Input: dimensioned drawing with shaded views. Units: mm. Origin: part minimum x, y, z. Coordinates: 2 decimals unless noted, no trailing zeros. Order: outer loops, then holes, each group sorted by start corner. A loop starts at its lowest first (then second) coordinate and runs counter-clockwise, first axis right, second up. Notation, with made-up numbers: (34.25, -3) -> (44.25, -3) arc R21 cw to (44.25, 16) -> close; hole circle Ø1 at (-1, 64.5). An arc over 180 degrees is marked (long way). Put each result on its own line as item: value.
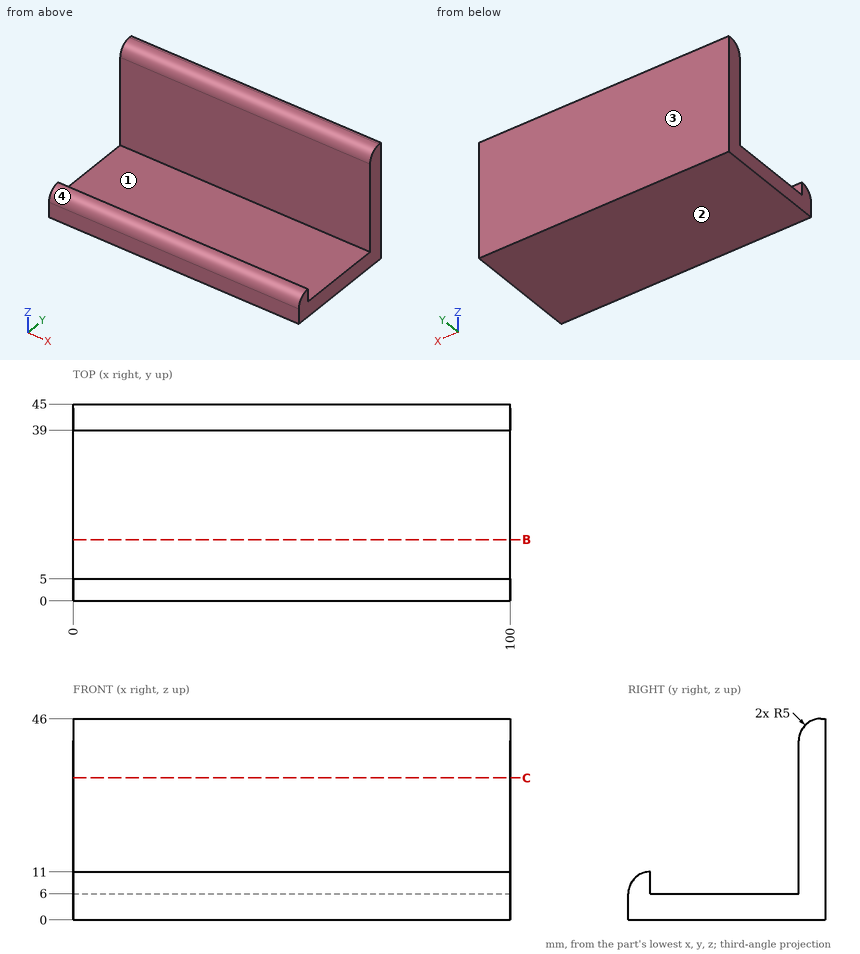
1. Cut plane C-C on z = 32.5. Output: boundary loops of the cut face in (x, y).
Numbers:
outline: (0, 39) -> (100, 39) -> (100, 45) -> (0, 45) -> close
2. Cut plane B-B on y = 14. Output: boundary loops of the cut face in (x, z).
Numbers:
outline: (0, 0) -> (100, 0) -> (100, 6) -> (0, 6) -> close
3. Ray query, line 1 along Z through (x, y) = (56.5, 18); line 2 along Y through (x, z) = (46, 14); line 3 along Z through (x, y) = (5.5, 41). Return the intervals inside material, ascending.
Numbers:
line 1: z = 0 to 6
line 2: y = 39 to 45
line 3: z = 0 to 45
4. First-contact query: pin 1 (1.5 mm diameter, centred on x = 31, z = 10.5, fed in from -Y); pin 2 (8 mm diameter, centred on x = 13, z = 10.5, fed in from -Y); pin 3 (2 mm diameter, centred on y = 37, z = 12, fed in from -X); pin 4 (2 mm diameter, centred on x = 58.5, y = 24.5, fed in from +Z). Flat tips, straight axial feed; report the tip coordinate or a pass-through.
Numbers:
pin 1: stops at y = 1.69
pin 2: stops at y = 0.03
pin 3: passes through
pin 4: stops at z = 6
5. Pull-direction query (Y, two-part tool) for the marked faces 1, 2, 3 and 4; classes: pulls with the +Y half, pulls with the -Y half, needs draft (parallel to the pull), parting line crosses it, or undercut.
Numbers:
face 1: undercut
face 2: needs draft
face 3: pulls with the +Y half
face 4: pulls with the -Y half
